```python
from build123d import *

# Parameters (mm, degrees)
F0_R     = 45
F0_R_2   = 7
F1_DEPTH = 3
F2_D     = 3.3
F3_D     = 3.3


with BuildPart() as f1:
    # F0 (on Front) → F1 (new body)
    with BuildSketch(Plane.XZ):
        Circle(F0_R)
        Circle(F0_R_2, mode=Mode.SUBTRACT)
    extrude(amount=-F1_DEPTH)

    # F2 (through all)
    with Locations(Plane.XZ):
        with Locations((-21.2132034356, 28.2842712475), (-28.2842712475, 21.2132034356), (-13.88829571, -32.5133086946), (-4.2290374471, -35.1014991456), (35.1014991456, 4.2290374471), (32.5133086946, 13.88829571)):
            Hole(F2_D / 2)

    # F3 (through all)
    with Locations(Plane.XZ):
        with Locations((0, 12.5), (0, -12.5)):
            Hole(F3_D / 2)


solid = f1.part
```
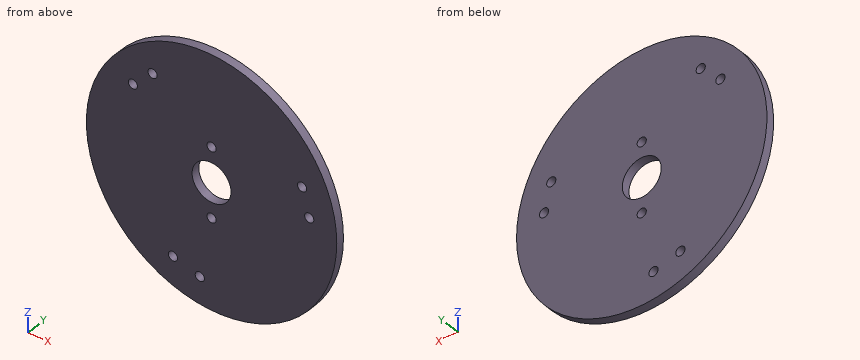
Geometry check sheet. Reference: the model listing, model coordinates, mm. Coordinates: 2 decimals unless noted, no trailing zeros. Loops run counter-clockwise (first coordinate to the right, second up) from the corner with the lowest first, then second, coordinate; pieces in that order, holes last. Notation, with made-up numbers: (-37, 12) - (-31, 12) arc R21 ccw to (-31, 47) - close; hole circle Ø8 at (-34.75, 73.5). An arc over 180 degrees is marked (long way). One line per item, written item: value. Start each with the question number.
(1) Depth check by flat-ended pin: P1, Ø1.5, axis at y = 0.5, z = -28.5, coming from the -X side. Enter the tip coordinate at first touch or a pass-through.
(2) Cross-section at D-D on x = -14. Enter the section's corners in (y, z).
(3) Cross-section at C-C on y = 1.4. Count the separate pieces of the cut face and the enclosed holes in it, plus the area to 3 significant figures.
(4) Cross-section at B-B on z = 0. Enter the section's corners in (x, y), plus the area to 3 significant figures.
(5) Cross-section at A-A on x = 0. Enter the section's corners in (y, z).
(6) Material ranges on line 1 (Z direction, x = 0, y = 0.8); line 2 (X direction, y = 2, z = 14); line 3 (X direction, y = 2.65, z = 5.5), recorded low to high. Write a range as [from, to].
Results below:
1. P1: stops at x = -35.43
2. outline: (0, -42.77) - (3, -42.77) - (3, -34.16) - (0, -34.16) - close; (0, -30.87) - (3, -30.87) - (3, 42.77) - (0, 42.77) - close
3. separate pieces: 1
3. enclosed holes: 9
3. area: 6,140 mm2
4. outline: (-45, 0) - (-7, 0) - (-7, 3) - (-45, 3) - close; (7, 0) - (45, 0) - (45, 3) - (7, 3) - close
4. area: 228 mm2
5. outline: (0, -45) - (3, -45) - (3, -14.15) - (0, -14.15) - close; (0, -10.85) - (3, -10.85) - (3, -7) - (0, -7) - close; (0, 7) - (3, 7) - (3, 10.85) - (0, 10.85) - close; (0, 14.15) - (3, 14.15) - (3, 45) - (0, 45) - close
6. line 1: z = [-45, -14.15], [-10.85, -7], [7, 10.85], [14.15, 45]
6. line 2: x = [-42.77, -0.69], [0.69, 30.87], [34.16, 42.77]
6. line 3: x = [-44.66, -4.33], [4.33, 34.05], [36.15, 44.66]
